from build123d import *

# Parameters (mm, degrees)
SKETCH1_W           = 50
SKETCH1_H           = 51.5
BOSS_EXTRUDE1_DEPTH = 3
SKETCH2_W           = 50
SKETCH2_H           = 3
BOSS_EXTRUDE2_DEPTH = 51
SKETCH3_R           = 11.05
SKETCH3_R_2         = 1.6
CUT_EXTRUDE1_DEPTH  = 90.823437921
CUT_EXTRUDE2_DEPTH  = 89.137676393
CHAMFER1_SIZE       = 5
FILLET1_R           = 7
FILLET2_R           = 2


with BuildPart() as part:
    # Sketch1 → Boss-Extrude1 (new body)
    with BuildSketch(Plane.XY):
        with Locations((25, 25.75)):
            Rectangle(SKETCH1_W, SKETCH1_H)
    extrude(amount=BOSS_EXTRUDE1_DEPTH)

    # Sketch2 → Boss-Extrude2 (add)
    with BuildSketch(Plane.XY.offset(3)):
        with Locations((25, 1.5)):
            Rectangle(SKETCH2_W, SKETCH2_H)
    extrude(amount=BOSS_EXTRUDE2_DEPTH)

    # Sketch3 → Cut-Extrude1 (cut, through all)
    with BuildSketch(Plane(origin=(0, 0, 0), x_dir=(-1, 0, 0), z_dir=(0, 0, -1))):
        with Locations((-25, 30)):
            Circle(SKETCH3_R)
        with Locations((-40.5, 45.5)):
            Circle(SKETCH3_R_2)
        with Locations((-9.5, 45.5)):
            Circle(SKETCH3_R_2)
        with Locations((-9.5, 14.5)):
            Circle(SKETCH3_R_2)
        with Locations((-40.5, 14.5)):
            Circle(SKETCH3_R_2)
    extrude(amount=-CUT_EXTRUDE1_DEPTH, mode=Mode.SUBTRACT)

    # Sketch4 → Cut-Extrude2 (cut, through all)
    with BuildSketch(Plane(origin=(0, 3, 0), x_dir=(1, 0, 0), z_dir=(0, 1, 0))):
        with BuildLine():
            Line((12.5, -13), (12.5, -42))
            ThreePointArc((12.5, -42), (10, -44.5), (7.5, -42))
            Line((7.5, -42), (7.5, -13))
            ThreePointArc((7.5, -13), (10, -10.5), (12.5, -13))
        make_face()
        with BuildLine():
            Line((37.5, -42), (37.5, -13))
            ThreePointArc((37.5, -13), (40, -10.5), (42.5, -13))
            Line((42.5, -13), (42.5, -42))
            ThreePointArc((42.5, -42), (40, -44.5), (37.5, -42))
        make_face()
    extrude(amount=-CUT_EXTRUDE2_DEPTH, mode=Mode.SUBTRACT)

    # Chamfer1
    chamfer1_edges = [part.edges().sort_by_distance(p)[0] for p in [
        (0, 1.5, 54),
        (50, 1.5, 54),
        (0, 51.5, 1.5),
        (50, 51.5, 1.5),
    ]]
    chamfer(chamfer1_edges, length=CHAMFER1_SIZE)

    # Fillet1
    fillet1_edges = [part.edges().sort_by_distance(p)[0] for p in [
        (25, 0, 0),
    ]]
    fillet(fillet1_edges, radius=FILLET1_R)

    # Fillet2
    fillet2_edges = [part.edges().sort_by_distance(p)[0] for p in [
        (25, 3, 3),
    ]]
    fillet(fillet2_edges, radius=FILLET2_R)


solid = part.part
Could you check a few things on this model? Use its own coordinates, in mm. A direction names the side the tool comes from. Give positions to 0.01 mm unless a question says otherwise; leave off trailing zeros. Write each loop counter-clockwise with the first axis right and the second up, starting at its lowest first coordinate (ties: lowest second). Pieces come first, ordered by that corner, then holes. Notation, with made-up numbers: (-5.75, 1) -> (14.25, 1) arc R12 cw to (14.25, 9) -> close; hole circle Ø8 at (66, 59.5). An arc over 180 degrees is marked (long way). Answer as a JSON object with one key per item and string values.
Q1. Suppose I cut it at A-A on z = 14.5. Write out the boundary of the cut face in (x, y).
Taken from the geometry:
{"outline": "(0, 0) -> (7.5, 0) -> (7.5, 3) -> (0, 3) -> close; (12.5, 0) -> (37.5, 0) -> (37.5, 3) -> (12.5, 3) -> close; (42.5, 0) -> (50, 0) -> (50, 3) -> (42.5, 3) -> close"}
Q2. Please list where these lines run through material, in increasing order: L1, parallel to Y at x = 40.5, z = 2.05; L2, parallel to Y at x = 19.5, z = 7.5; L3, parallel to Y at x = 40.5, z = 1.85.
Taken from the geometry:
{"L1": "y = 2.05 to 12.9, 16.1 to 43.9, 47.1 to 51.5", "L2": "y = 0 to 3", "L3": "y = 2.26 to 12.9, 16.1 to 43.9, 47.1 to 51.5"}
Q3. Suppose I cut it at C-C on x = 9.5. Write out the boundary of the cut face in (y, z), then the cut area to 3 significant figures.
Taken from the geometry:
{"outline": "(0, 7) arc R7 ccw to (7, 0) -> (12.9, 0) -> (12.9, 3) -> (5, 3) arc R2 cw to (3, 5) -> (3, 10.55) -> (0, 10.55) -> close; (0, 44.45) -> (3, 44.45) -> (3, 54) -> (0, 54) -> close; (16.1, 0) -> (43.9, 0) -> (43.9, 3) -> (16.1, 3) -> close; (47.1, 0) -> (51.5, 0) -> (51.5, 3) -> (47.1, 3) -> close", "area": "177 mm²"}
Q4. Which directions (+Z, -Z, +X, -X, +Y, -Y) give clear straight access to the entire face, cutting with the end or side of a thin tool? Please do faces 4 (the flat face through (48, 1, 51)), 5 (the flat face through (25, 3, 29)), 6 (the flat face through (12.5, 2, 27)).
Taken from the geometry:
{"face 4": "+Z, +X, +Y, -Y", "face 5": "+Z, +X, -X, +Y", "face 6": "+Y, -Y"}
Q5. Will these pins go through, and if not, where does the flat tip stop? pin 1 Ø3.5 at (x, y) = (40.5, 14.5) entering from +Z; pin 2 Ø1.5 at (x, z) = (44.5, 11) entering from +Y.
Taken from the geometry:
{"pin 1": "stops at z = 3", "pin 2": "stops at y = 3"}
Q6. We'd pull the mould along X, two halves only. Please class faces 1 (the cylindrical face through (25.35, 3.57, 3.6)), 2 (the cylindrical face through (14.46, 33.32, 1.48)), 3 (the flat face through (2.5, 49, 1.5)): released by +X, released by -X, zero draft, split by the parting line, or undercut.
Taken from the geometry:
{"face 1": "zero draft", "face 2": "undercut", "face 3": "released by -X"}
Q7. Suppose I cut it at D-D on y = 40. Write out the boundary of the cut face in (x, z).
Taken from the geometry:
{"outline": "(0, 0) -> (20.3, 0) -> (20.3, 3) -> (0, 3) -> close; (29.7, 0) -> (50, 0) -> (50, 3) -> (29.7, 3) -> close"}
Q8. Suppose I cut it at B-B on y = 14.5. Write out the boundary of the cut face in (x, z).
Taken from the geometry:
{"outline": "(0, 0) -> (7.9, 0) -> (7.9, 3) -> (0, 3) -> close; (11.1, 0) -> (38.9, 0) -> (38.9, 3) -> (11.1, 3) -> close; (42.1, 0) -> (50, 0) -> (50, 3) -> (42.1, 3) -> close"}
